Job drawing, mm, ordinate dimensions from the low corner. One solid piece. Give positions to 0.01 mm unless a question says otherwise; leave off trailing zeros. Order: outer loops, then holes, each group sorted by start corner. A loop starts at its lowest first (then second) coordinate and runs counter-clockwise, first axis right, second up.
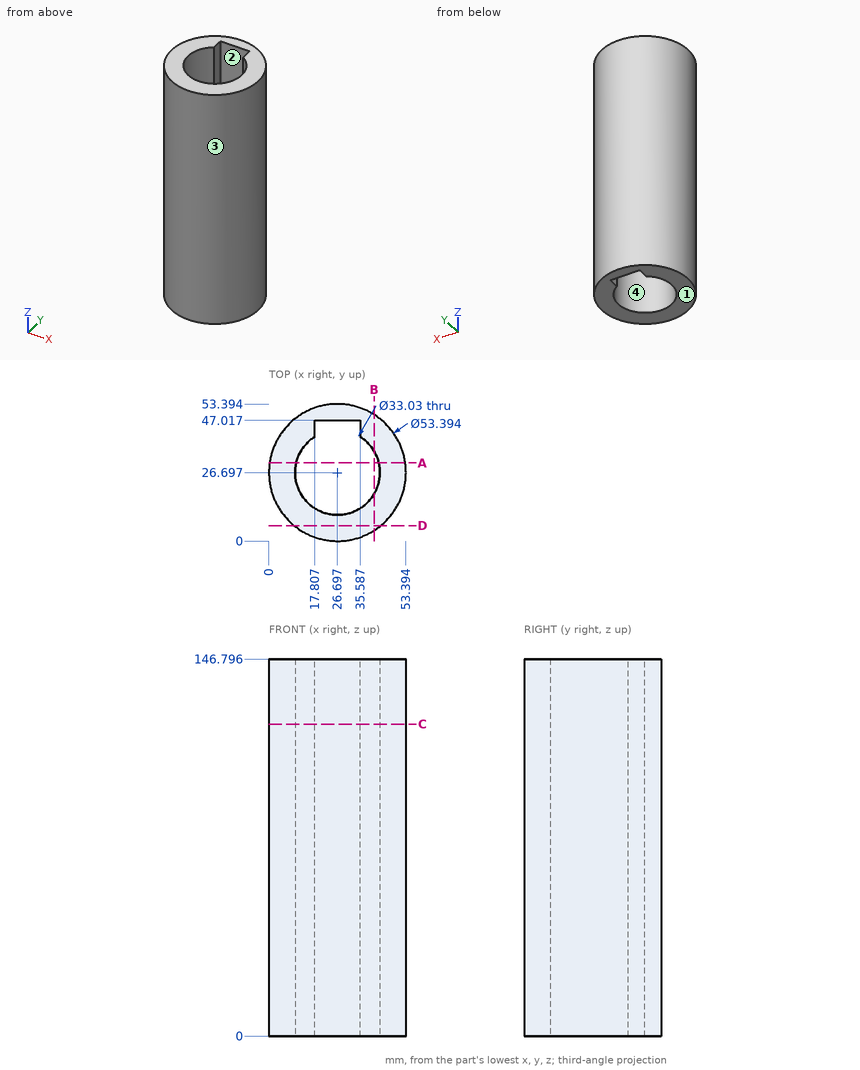
Item 1: Pull direction X, two halves, no side cores. Call the marked faces 1, 2, 3 and 4: released by +X, released by -X, zero draft, split by the parting line, or undercut.
Item 2: Band-saw the part on B-B on x = 41. List the corners of the cut face in (y, z) (1 decimal).
Item 3: Drop flat-ended pins along their axis: P1, Ø3, axis at x = 31, z = 53.5, coming from the -Y side; P2, Ø19.5, axis at x = 26, z = 37, coming from the -Y side; P3, Ø5, axis at y = 42.5, z = 82, coming from the +X side; P4, Ø1.5, axis at x = 6.5, y = 7, coming from the -Z side. Give the stop position or say it passes through.
Item 4: Band-saw the part on A-A on y = 30.5. List the corners of the cut face in (x, z) (1 decimal).
Item 5: Band-saw the part on D-D on y = 6. List the corners of the cut face in (x, z), plus the area to 3 significant figures.
Item 6: Drill centre lines: probe 1 along Y at (x, z) = (26, 102) (1 decimal); probe 2 along X at (y, z) = (26.5, 63.5); probe 3 along X at (y, z) = (45, 20) (1 decimal). Where is each one in solid material? Low to high.
Item 7: Band-saw the part on C-C on z = 121.5. List the corners of the cut face in (x, y) (1 decimal), plus the area to 3 significant figures.
Working result:
1. face 1: zero draft
1. face 2: undercut
1. face 3: split by the parting line
1. face 4: undercut
2. outline: (4.2, 0) - (18.4, 0) - (18.4, 146.8) - (4.2, 146.8) - close; (35, 0) - (49.2, 0) - (49.2, 146.8) - (35, 146.8) - close
3. P1: stops at y = 0.15
3. P2: stops at y = 0
3. P3: stops at x = 49.84
3. P4: passes through
4. outline: (0.3, 0) - (10.6, 0) - (10.6, 146.8) - (0.3, 146.8) - close; (42.8, 0) - (53.1, 0) - (53.1, 146.8) - (42.8, 146.8) - close
5. outline: (9.83, 0) - (43.56, 0) - (43.56, 146.8) - (9.83, 146.8) - close
5. area: 4,950 mm2
6. probe 1: y = 0 to 10.2, 47 to 53.4
6. probe 2: x = 0 to 10.18, 43.21 to 53.39
6. probe 3: x = 7.3 to 17.8, 35.6 to 46.1
7. outline: circle Ø53.4 at (26.7, 26.7); hole (17.8, 40.6) arc R16.5 ccw (long way) to (35.6, 40.6) - (35.6, 47) - (17.8, 47) - close
7. area: 1,300 mm2
